Here's how the part is built. I have some questions about the finished solid (model axes, mm). A direction names the side the tool comes from. Give positions to 0.01 mm unless a question says otherwise; leave off trailing zeros. Loops run counter-clockwise (first coordinate to the right, second up) from the corner with the lowest first, then second, coordinate; pieces in that order, holes last. Notation, with made-up numbers: (78.25, -39) - (89.25, -39) arc R10 ccw to (89.25, -35) - close; hole circle Ø8 at (77.5, 51). An arc over 180 degrees is marked (long way). Use a Markdown table: item, result.
from build123d import *

# Parameters (mm, degrees)
SKETCH_R           = 20
PAD_DEPTH          = 8
POCKET_DEPTH       = 8.001
SKETCH003_R        = 3.5
POCKET001_DEPTH    = 7
POLARPATTERN_COUNT = 5
SKETCH005_R        = 1.995724
POCKET002_DEPTH    = 0.5
SKETCH007_R        = 17.476315
SKETCH007_R_2      = 3.403878
PAD001_DEPTH       = 1
POCKET003_DEPTH    = 8.001


with BuildPart() as part:
    # Sketch → Pad (new body)
    with BuildSketch(Plane.XY):
        Circle(SKETCH_R)
    extrude(amount=PAD_DEPTH)

    # Sketch001 (on Face3 of Pad) → Pocket (cut, through all)
    with BuildSketch(Plane.XY.offset(8)):
        with BuildLine():
            ThreePointArc((1.101147, -2.25), (0, 2.505), (-1.101147, -2.25))
            Line((-1.101147, -2.25), (1.101147, -2.25))
        make_face()
    extrude(amount=-POCKET_DEPTH, mode=Mode.SUBTRACT)

    # Sketch002 → Groove (revolve, cut)
    with BuildSketch(Plane.XZ):
        Polygon((19.5, 6.5), (19.5, 1), (23, 1), (23, 10), align=None)
    revolve(axis=Axis((0, 0, 0), (0, 0, 1)), mode=Mode.SUBTRACT)

    # Sketch003 (on Face3 of Groove) → Pocket001 (cut)
    with BuildSketch(Plane.XY.offset(8)):
        with Locations((0, 13)):
            Circle(SKETCH003_R)
    pocket001 = extrude(amount=-POCKET001_DEPTH, mode=Mode.SUBTRACT)

    # PolarPattern: Pocket001 ×5 about axis
    polarpattern_axis = Axis((0, 0, 8), (0, 0, 1))
    for i in range(1, POLARPATTERN_COUNT):
        add(pocket001.rotate(polarpattern_axis, i * 360 / POLARPATTERN_COUNT), mode=Mode.SUBTRACT)

    # Sketch005 (on Face3 of PolarPattern) → Pocket002 (cut)
    with BuildSketch(Plane.XY.offset(8)):
        with Locations((-5.881012, 7.168965)):
            Circle(SKETCH005_R)
    extrude(amount=-POCKET002_DEPTH, mode=Mode.SUBTRACT)

    # Sketch007 (on Face3 of Pocket002) → Pad001 (join)
    with BuildSketch(Plane.XY.offset(8)):
        Circle(SKETCH007_R)
        Circle(SKETCH007_R_2, mode=Mode.SUBTRACT)
    extrude(amount=-PAD001_DEPTH)

    # Sketch008 (on Face5 of Pad001) → Pocket003 (cut, through all)
    with BuildSketch(Plane.XY.offset(8)):
        Polygon((0, 0), (-0.444954, 0.22807), (10.469651, 21.521968), (11.359559, 21.065828), (0.444954, -0.22807), align=None)
    extrude(amount=-POCKET003_DEPTH, mode=Mode.SUBTRACT)


solid = part.part
(1) Will these pins go through, and if not, where does the flat tip stop? pin 1 (4 mm diameter, centred on y = 6.5, z = 6, fed in from -X); pin 2 (2 mm diameter, centred on x = -14, z = 4.5, fed in from +Y); pin 3 (3 mm diameter, centred on y = 0.5, z = 3, fed in from -X).
A:
| item | result |
|---|---|
| pin 1 | x = -19.42 |
| pin 2 | y = 14.53 |
| pin 3 | x = -19.5 |
(2) Suppose I cut it at B-B on z = 1.75. Write out the boundary of the cut face in (x, y) (3 decimals), plus the area to 3 significant figures.
A:
| item | result |
|---|---|
| outline | (-1.101, -2.25) arc R2.505 cw to (0.675, 2.412) - (8.447, 17.576) arc R19.5 ccw (long way) to (9.337, 17.119) - (1.565, 1.956) arc R2.505 cw to (1.101, -2.25) - close; hole circle Ø7 at (-12.364, 4.017); hole circle Ø7 at (-7.641, -10.517); hole circle Ø7 at (0, 13); hole circle Ø7 at (7.641, -10.517); hole circle Ø7 at (12.364, 4.017) |
| area | 966 mm2 |
(3) Suppose I cut it at C-C on y = -11. Count the separate pieces of the cut face and the enclosed holes in it, plus the area to 3 significant figures.
A:
| item | result |
|---|---|
| separate pieces | 1 |
| enclosed holes | 2 |
| area | 177 mm2 |
(4) We'd pull the mould along Y, two halves only. Please class faces 4 (the face through (-19.2, -4.4, 1)), 5 (the face through (-9.35, 2.24, 4.04)), 6 (the face through (-8, -10, 7)): pulls with the +Y half, pulls with the -Y half, needs draft (parallel to the pull), parting line crosses it, or undercut.
A:
| item | result |
|---|---|
| face 4 | needs draft |
| face 5 | undercut |
| face 6 | undercut |
(5) Suppose I cut it at A-A on x = 0. Write out the boundary of the cut face in (y, z) (3 decimals), plus the area to 3 significant figures.
A:
| item | result |
|---|---|
| outline | (-20, 0) - (-2.25, 0) - (-2.25, 8) - (-20, 8) - (-20, 7) - (-19.5, 6.5) - (-19.5, 1) - (-20, 1) - close; (2.505, 0) - (20, 0) - (20, 1) - (19.5, 1) - (19.5, 6.5) - (20, 7) - (20, 8) - (2.505, 8) - close; hole (9.5, 1) - (16.5, 1) - (16.5, 7) - (9.5, 7) - close |
| area | 234 mm2 |
(6) On a 3-axis mill with a long thin cutter (end or side, diameter ignored), from which of +Z, -Z, +X, -X, +Y, -Y can I reach the whole of each face in a straight line? I mean faces 1 (the face through (12, 4, 7)), 2 (the face through (2.486, -0.309, 4.056)), 3 (the face through (0, -4, 0)). Say none if no direction works.
A:
| item | result |
|---|---|
| face 1 | none |
| face 2 | +Z, -Z |
| face 3 | -Z, +X, -X, +Y, -Y |
(7) If I drill on line 1 (Y direction, x = 0, z = 3.45) (3 decimals); line 2 (Z direction, x = -11, y = -10); line 3 (X direction, y = -10, z = 6.75), over which ranges is the centre line in solid material (lowest first)?
A:
| item | result |
|---|---|
| line 1 | -19.5 to -2.25, 2.505 to 9.5, 16.5 to 19.5 |
| line 2 | 0 to 1, 7 to 8 |
| line 3 | -17.03 to -11.1, -4.18 to 4.18, 11.1 to 17.03 |
